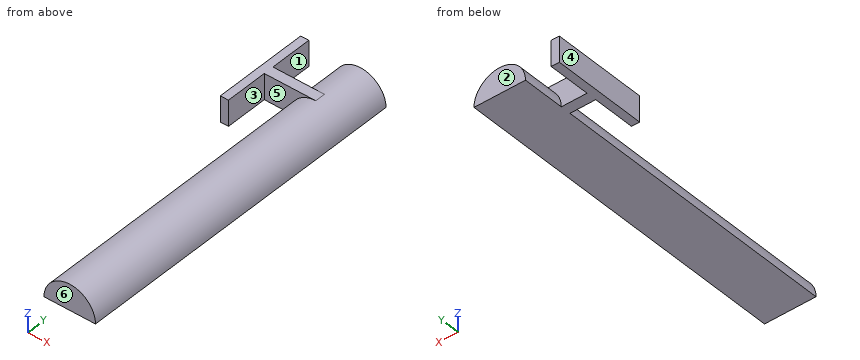
from build123d import *

# Parameters (mm, degrees)
F1_DEPTH = 170
F2_W     = 25.4
F2_H     = 5.08
F3_DEPTH = 12.7
F4_W     = 20.96
F4_H     = 12.7
F4_W_2   = 2.54
F5_DEPTH = 4


with BuildPart() as f1:
    # F0 (on Front) → F1 (new body)
    with BuildSketch(Plane.XZ):
        with BuildLine():
            Line((-12.7, 0), (12.7, 0))
            ThreePointArc((12.7, 0), (0, 12.7), (-12.7, 0))
        make_face()
    extrude(amount=F1_DEPTH)

    # F2 (on face) → F3 (join)
    with BuildSketch(Plane(origin=(0, 0, 0), x_dir=(1, 0, 0), z_dir=(0, 0, -1))):
        with Locations((-12.7, 23.5)):
            Rectangle(F2_W, F2_H)
    extrude(amount=-F3_DEPTH)

    # F4 (on face) → F5 (join)
    with BuildSketch(Plane(origin=(-25.4, 0, 0), x_dir=(0, -1, 0), z_dir=(-1, 0, 0))):
        with Locations((36.52, 6.35)):
            Rectangle(F4_W, F4_H)
        with Locations((10.48, 6.35)):
            Rectangle(F4_W, F4_H)
        with Locations((22.23, 6.35)):
            Rectangle(F4_W_2, F4_H)
        with Locations((24.77, 6.35)):
            Rectangle(F4_W_2, F4_H)
    extrude(amount=F5_DEPTH)


solid = f1.part
Build history of the part. All positions in model axes, mm. Face numbers are marked on the shaded views. A direction names the side the tool comes from. Give positions to 0.01 mm unless a question says otherwise; leave off trailing zeros. Order: outer loops, then holes, each group sorted by start corner. A loop starts at its lowest first (then second) coordinate and runs counter-clockwise, first axis right, second up. Notation, with made-up numbers: M -15.75,33.5 L 9.25,33.5 A6 ccw 9.25,44.5 Z; hole C 42,67 d7. An arc over 180 degrees is marked long. Use one line per item in the form item = value.
Q1. Which spindle directions (+Z, -Z, +X, -X, +Y, -Y) get a long thin tool onto all of the face, cutting with end or side? Do the marked faces 1, 2 and 3. Say none if no direction does.
Conclusion:
face_1 = +Z, -Z, +Y
face_2 = +Z, -Z, +X, -X, +Y
face_3 = +Z, -Z, -Y
Q2. Pull direction X, two halves, no side cores. Call the marked faces 4, 5 and 6: released by +X, released by -X, zero draft, split by the parting line, or undercut.
Conclusion:
face_4 = released by -X
face_5 = undercut
face_6 = zero draft
Q3. Wall check: probe 1 along Y at (x, z) = (-11.5, 6.5); probe 2 along X at (y, z) = (-11, 2.5); probe 3 along X at (y, z) = (-15, 11.5). Give the ranges that are in metal, low to high.
Conclusion:
probe_1 = -26.04 to -20.96
probe_2 = -29.4 to -25.4, -12.45 to 12.45
probe_3 = -29.4 to -25.4, -5.39 to 5.39
Q4. Slice it at D-D, the plane y = -89. Write the cut outline in (x, z).
Conclusion:
outline = M -12.7,0 L 12.7,0 A12.7 ccw Z
Q5. Pin check, flat tips, straight feed: P1, Ø1.5, axis at y = -152, z = 11, coming from the +X side; P2, Ø3, axis at y = -80.5, z = 7.5, coming from the +X side; P3, Ø1.5, axis at x = -19, z = 7, coming from the +Y side. Stop position of each tip, or through.
Conclusion:
P1 = 7.5
P2 = 11.19
P3 = -20.96
Q6. Slice it at A-A, the plane y = -38. Write the cut outline in (x, z).
Conclusion:
outline = M -29.4,0 L -25.4,0 L -25.4,12.7 L -29.4,12.7 Z; M -12.7,0 L 12.7,0 A12.7 ccw Z
Q7. Slice it at B-B, the plane z = 10.5. Write the cut outline in (x, y).
Conclusion:
outline = M -29.4,-47 L -25.4,-47 L -25.4,-26.04 L -7.14,-26.04 L -7.14,-170 L 7.14,-170 L 7.14,0 L -7.14,0 L -7.14,-20.96 L -25.4,-20.96 L -25.4,0 L -29.4,0 Z
Q8. Slice it at C-C, the plane x = -8.5. Write the cut outline in (y, z).
Conclusion:
outline = M -170,0 L 0,0 L 0,9.44 L -20.96,9.44 L -20.96,12.7 L -26.04,12.7 L -26.04,9.44 L -170,9.44 Z
